Autodesk Inventor part; units mm, degrees
ref_plane "YZ Plane" through (0, 0, 0) normal (1, 0, 0) x (0, 1, 0)
ref_plane "XZ Plane" through (0, 0, 0) normal (0, 1, 0) x (-1, 0, 0)
ref_plane "XY Plane" through (0, 0, 0) normal (0, 0, 1) x (1, 0, 0)
ref_plane "Arbeitsebene1" through (-6.2499, 0, 0) normal (0, 0, 1) x (1, 0, 0)
sketch "Skizze1" plane through (-6.2499, 0, 0) normal (0, 0, 1) x (1, 0, 0)
  line L0 (21.2499, 26.0506) -> (21.2499, 58.2506)
  line L1 (21.2499, 58.2506) -> (-8.7501, 58.2506)
  line L2 (-8.7501, 58.2506) -> (-8.7501, 26.0506)
  line L3 (-8.7501, 26.0506) -> (21.2499, 26.0506)
  circle A0 centre (16.2499, 32.1506) radius 1.25
  circle A1 centre (-3.7501, 32.1506) radius 1.25
  circle A2 centre (-3.7501, 52.1506) radius 1.25
  circle A3 centre (16.2499, 52.1506) radius 1.25
  circle A4 centre (13.7499, 38.0506) radius 3.25
  circle A5 centre (13.7499, 46.2506) radius 3.25
  circle A6 centre (-1.2501, 38.0506) radius 3.25
  circle A7 centre (-1.2501, 46.2506) radius 3.25
  line L4 (-67.7501, 103.2266) -> (-67.7501, 101.9266) construction
  line L5 (-18.7501, 103.2266) -> (-67.7501, 103.2266) construction
  arc A8 (-15.2501, 99.7266) -> (-18.7501, 103.2266) centre (-18.7501, 99.7266) ccw construction
  line L6 (-15.2501, 22.1266) -> (-15.2501, 99.7266) construction
  arc A9 (-18.7501, 18.6266) -> (-15.2501, 22.1266) centre (-18.7501, 22.1266) ccw construction
  line L7 (-67.7501, 18.6266) -> (-18.7501, 18.6266) construction
  line L8 (-67.7501, 19.9266) -> (-67.7501, 18.6266) construction
  line L9 (-23.4028, 19.9266) -> (-67.7501, 19.9266) construction
  arc A10 (-23.4028, 19.9266) -> (-21.8472, 20.571) centre (-23.4028, 22.1266) ccw construction
  line L10 (-17.1945, 25.2237) -> (-21.8472, 20.571) construction
  arc A11 (-17.1945, 25.2237) -> (-16.5501, 26.7793) centre (-18.7501, 26.7793) ccw construction
  line L11 (-16.5501, 95.0739) -> (-16.5501, 26.7793) construction
  arc A12 (-16.5501, 95.0739) -> (-17.1945, 96.6296) centre (-18.7501, 95.0739) ccw construction
  line L12 (-21.8472, 101.2823) -> (-17.1945, 96.6296) construction
  arc A13 (-21.8472, 101.2823) -> (-23.4028, 101.9266) centre (-23.4028, 99.7266) ccw construction
  line L13 (-67.7501, 101.9266) -> (-23.4028, 101.9266) construction
  arc A14 (-18.7501, 18.2266) -> (-14.8501, 22.1266) centre (-18.7501, 22.1266) ccw construction
  line L14 (-14.8501, 22.1266) -> (-14.8501, 99.7266) construction
  line L15 (-18.7501, 103.6266) -> (-68.1501, 103.6266) construction
  line L16 (-68.1501, 103.6266) -> (-68.1501, 101.5266) construction
  line L17 (-68.1501, 101.5266) -> (-23.4028, 101.5266) construction
  arc A15 (-22.13, 100.9994) -> (-23.4028, 101.5266) centre (-23.4028, 99.7266) ccw construction
  line L18 (-22.13, 100.9994) -> (-17.4773, 96.3467) construction
  arc A16 (-16.9501, 95.0739) -> (-17.4773, 96.3467) centre (-18.7501, 95.0739) ccw construction
  line L19 (-16.9501, 95.0739) -> (-16.9501, 26.7793) construction
  arc A17 (-17.4773, 25.5065) -> (-16.9501, 26.7793) centre (-18.7501, 26.7793) ccw construction
  line L20 (-17.4773, 25.5065) -> (-22.13, 20.8538) construction
  arc A18 (-23.4028, 20.3266) -> (-22.13, 20.8538) centre (-23.4028, 22.1266) ccw construction
  line L21 (-23.4028, 20.3266) -> (-68.1501, 20.3266) construction
  line L22 (-68.1501, 20.3266) -> (-68.1501, 18.2266) construction
  line L23 (-68.1501, 18.2266) -> (-18.7501, 18.2266) construction
  arc A19 (-18.7501, 18.2266) -> (-14.8501, 22.1266) centre (-18.7501, 22.1266) ccw construction
  line L24 (-14.8501, 22.1266) -> (-14.8501, 99.7266) construction
  arc A20 (-14.8501, 99.7266) -> (-18.7501, 103.6266) centre (-18.7501, 99.7266) ccw construction
  line L25 (-89.5501, 101.9266) -> (-89.5501, 103.2266) construction
  line L26 (-138.8501, 101.9266) -> (-89.5501, 101.9266) construction
  arc A21 (-138.8501, 101.9266) -> (-140.7501, 100.0266) centre (-138.8501, 100.0266) ccw construction
  line L27 (-140.7501, 21.8266) -> (-140.7501, 100.0266) construction
  arc A22 (-140.7501, 21.8266) -> (-138.8501, 19.9266) centre (-138.8501, 21.8266) ccw construction
  line L28 (-89.5501, 19.9266) -> (-138.8501, 19.9266) construction
  line L29 (-89.5501, 18.6266) -> (-89.5501, 19.9266) construction
  line L30 (-138.5501, 18.6266) -> (-89.5501, 18.6266) construction
  arc A23 (-142.0501, 22.1266) -> (-138.5501, 18.6266) centre (-138.5501, 22.1266) ccw construction
  line L31 (-142.0501, 99.7266) -> (-142.0501, 22.1266) construction
  arc A24 (-138.5501, 103.2266) -> (-142.0501, 99.7266) centre (-138.5501, 99.7266) ccw construction
  line L32 (-89.5501, 103.2266) -> (-138.5501, 103.2266) construction
  arc A25 (-138.5501, 103.6266) -> (-142.4501, 99.7266) centre (-138.5501, 99.7266) ccw construction
  line L33 (-142.4501, 99.7266) -> (-142.4501, 22.1266) construction
  arc A26 (-142.4501, 22.1266) -> (-138.5501, 18.2266) centre (-138.5501, 22.1266) ccw construction
  line L34 (-138.5501, 18.2266) -> (-89.1501, 18.2266) construction
  line L35 (-89.1501, 18.2266) -> (-89.1501, 20.3266) construction
  line L36 (-89.1501, 20.3266) -> (-138.8501, 20.3266) construction
  arc A27 (-140.3501, 21.8266) -> (-138.8501, 20.3266) centre (-138.8501, 21.8266) ccw construction
  line L37 (-140.3501, 21.8266) -> (-140.3501, 100.0266) construction
  arc A28 (-138.8501, 101.5266) -> (-140.3501, 100.0266) centre (-138.8501, 100.0266) ccw construction
  line L38 (-138.8501, 101.5266) -> (-89.1501, 101.5266) construction
  line L39 (-89.1501, 101.5266) -> (-89.1501, 103.6266) construction
  line L40 (-89.1501, 103.6266) -> (-138.5501, 103.6266) construction
  line L41 (-68.6501, 104.1266) -> (-18.7501, 104.1266)
  arc A29 (-14.3501, 99.7266) -> (-18.7501, 104.1266) centre (-18.7501, 99.7266) ccw
  line L42 (-14.3501, 99.7266) -> (-14.3501, 22.1266)
  arc A30 (-18.7501, 17.7266) -> (-14.3501, 22.1266) centre (-18.7501, 22.1266) ccw
  line L43 (-18.7501, 17.7266) -> (-68.6501, 17.7266)
  line L44 (-68.6501, 17.7266) -> (-68.6501, 20.8266)
  line L45 (-68.6501, 20.8266) -> (-23.4028, 20.8266)
  arc A31 (-23.4028, 20.8266) -> (-22.4836, 21.2074) centre (-23.4028, 22.1266) ccw
  line L46 (-22.4836, 21.2074) -> (-17.8309, 25.8601)
  arc A32 (-17.8309, 25.8601) -> (-17.4501, 26.7793) centre (-18.7501, 26.7793) ccw
  line L47 (-17.4501, 26.7793) -> (-17.4501, 95.0739)
  arc A33 (-17.4501, 95.0739) -> (-17.8309, 95.9932) centre (-18.7501, 95.0739) ccw
  line L48 (-17.8309, 95.9932) -> (-22.4836, 100.6459)
  arc A34 (-22.4836, 100.6459) -> (-23.4028, 101.0266) centre (-23.4028, 99.7266) ccw
  line L49 (-23.4028, 101.0266) -> (-68.6501, 101.0266)
  line L50 (-68.6501, 101.0266) -> (-68.6501, 104.1266)
  arc A35 (-138.5501, 104.1266) -> (-142.9501, 99.7266) centre (-138.5501, 99.7266) ccw
  line L51 (-142.9501, 99.7266) -> (-142.9501, 22.1266)
  arc A36 (-142.9501, 22.1266) -> (-138.5501, 17.7266) centre (-138.5501, 22.1266) ccw
  line L52 (-138.5501, 17.7266) -> (-88.6501, 17.7266)
  line L53 (-88.6501, 17.7266) -> (-88.6501, 20.8266)
  line L54 (-88.6501, 20.8266) -> (-138.8501, 20.8266)
  arc A37 (-139.8501, 21.8266) -> (-138.8501, 20.8266) centre (-138.8501, 21.8266) ccw
  line L55 (-139.8501, 21.8266) -> (-139.8501, 100.0266)
  arc A38 (-138.8501, 101.0266) -> (-139.8501, 100.0266) centre (-138.8501, 100.0266) ccw
  line L56 (-138.8501, 101.0266) -> (-88.6501, 101.0266)
  line L57 (-88.6501, 101.0266) -> (-88.6501, 104.1266)
  line L58 (-88.6501, 104.1266) -> (-138.5501, 104.1266)
  line L59 (-68.6501, 104.1266) -> (-88.6501, 104.1266)
  line L60 (-88.6501, 17.7266) -> (-68.6501, 17.7266)
  line L61 (-94.9, 12.7266) -> (-138.5501, 12.7266)
  arc A39 (-147.9501, 22.1266) -> (-138.5501, 12.7266) centre (-138.5501, 22.1266) ccw
  line L62 (-147.9501, 22.1266) -> (-147.9501, 99.7266)
  arc A40 (-138.5501, 109.1266) -> (-147.9501, 99.7266) centre (-138.5501, 99.7266) ccw
  line L63 (-138.5501, 109.1266) -> (-94.9, 109.1266)
  line L64 (-74.9, 12.7266) -> (-18.7501, 12.7266)
  arc A41 (-18.7501, 12.7266) -> (-9.3501, 22.1266) centre (-18.7501, 22.1266) ccw
  line L65 (-9.3501, 22.1266) -> (-9.3501, 99.7266)
  arc A42 (-9.3501, 99.7266) -> (-18.7501, 109.1266) centre (-18.7501, 99.7266) ccw
  line L66 (-18.7501, 109.1266) -> (-74.9, 109.1266)
  line L67 (-94.9, 12.7266) -> (-74.9, 12.7266)
  line L68 (-74.9, 109.1266) -> (-94.9, 109.1266)
  line L69 (-8.7501, 58.2506) -> (-9.3501, 58.2506)
  line L70 (-8.7501, 26.0506) -> (-9.3501, 26.0506)
  point P0 (6.2499, 0)
  point P1 (-12.4751, 58.2506)
  point P2 (-12.4751, 26.0506)
  point P3 (-12.4751, 26.0506)
  dimension "d0" = 0
  dimension "d1" = 0
  dimension "d2" = 0.5
  dimension "d3" = 0.5
  dimension "d4" = 5
  dimension "d5" = 5
extrude "Extrusion1" add sketch "Skizze1" along normal blind 10 contours L3 L2 L1 L0 | L70 L65 L69 L2 | L65 A41 L64 L67 L61 A39 L62 A40 L63 L68 L66 A42 | A4 | A5 | A6 | A7
sketch "Skizze3" plane through (-6.2499, 0, 0) normal (0, 0, -1) x (-1, 0, 0)
  line L0 (9.3501, 26.0506) -> (-21.2499, 26.0506)
  line L1 (9.3501, 22.1266) -> (9.3501, 26.0506)
  arc A0 (9.3501, 22.1266) -> (18.7501, 12.7266) centre (18.7501, 22.1266) ccw
  line L2 (138.5501, 12.7266) -> (18.7501, 12.7266)
  arc A1 (138.5501, 12.7266) -> (147.9501, 22.1266) centre (138.5501, 22.1266) ccw
  line L3 (147.9501, 99.7266) -> (147.9501, 22.1266)
  arc A2 (147.9501, 99.7266) -> (138.5501, 109.1266) centre (138.5501, 99.7266) ccw
  line L4 (18.7501, 109.1266) -> (138.5501, 109.1266)
  arc A3 (18.7501, 109.1266) -> (9.3501, 99.7266) centre (18.7501, 99.7266) ccw
  line L5 (9.3501, 58.2506) -> (9.3501, 99.7266)
  line L6 (-21.2499, 58.2506) -> (9.3501, 58.2506)
  line L7 (-21.2499, 26.0506) -> (-21.2499, 58.2506)
  circle A4 centre (-16.2499, 32.1506) radius 1.25
  circle A5 centre (3.7501, 32.1506) radius 1.25
  circle A6 centre (3.7501, 52.1506) radius 1.25
  circle A7 centre (-16.2499, 52.1506) radius 1.25
  line L8 (18.7501, 17.7266) -> (138.5501, 17.7266)
  arc A8 (14.3501, 22.1266) -> (18.7501, 17.7266) centre (18.7501, 22.1266) ccw
  line L9 (14.3501, 99.7266) -> (14.3501, 22.1266)
  arc A9 (18.7501, 104.1266) -> (14.3501, 99.7266) centre (18.7501, 99.7266) ccw
  line L10 (138.5501, 104.1266) -> (18.7501, 104.1266)
  arc A10 (142.9501, 99.7266) -> (138.5501, 104.1266) centre (138.5501, 99.7266) ccw
  line L11 (142.9501, 22.1266) -> (142.9501, 99.7266)
  arc A11 (138.5501, 17.7266) -> (142.9501, 22.1266) centre (138.5501, 22.1266) ccw
  arc A12 (141.4501, 99.7266) -> (138.5501, 102.6266) centre (138.5501, 99.7266) ccw
  line L12 (138.5501, 102.6266) -> (18.7501, 102.6266)
  arc A13 (18.7501, 102.6266) -> (15.8501, 99.7266) centre (18.7501, 99.7266) ccw
  line L13 (15.8501, 99.7266) -> (15.8501, 22.1266)
  arc A14 (15.8501, 22.1266) -> (18.7501, 19.2266) centre (18.7501, 22.1266) ccw
  line L14 (18.7501, 19.2266) -> (138.5501, 19.2266)
  arc A15 (138.5501, 19.2266) -> (141.4501, 22.1266) centre (138.5501, 22.1266) ccw
  line L15 (141.4501, 22.1266) -> (141.4501, 99.7266)
  point P0 (-6.2499, 0)
  dimension "d11" = 1.5
extrude "Extrusion3" add sketch "Skizze3" against normal blind 1 contours A8 L9 A9 L10 A10 L11 A11 L8
sketch "Skizze4" plane through (-144.8, 12.7266, 0) normal (0, -1, 0) x (1, 0, 0)
  line L0 (0, 10) -> (119.8, 10)
  line L1 (19.9, 10) -> (99.9, 10) construction
  line L2 (0, 10) -> (119.8, 10)
  line L3 (19.9, 7.5) -> (99.9, 7.5)
  line L4 (99.9, 12.5) -> (19.9, 12.5)
  arc A0 (19.9, 12.5) -> (19.9, 7.5) centre (19.9, 10) ccw
  arc A1 (99.9, 7.5) -> (99.9, 12.5) centre (99.9, 10) ccw
  point P0 (144.8, 0)
  point P1 (59.9, 10)
  point P2 (102.4, 10)
  point P3 (17.4, 10)
  dimension "d14" = 40
  dimension "d18" = 5
extrude "Extrusion4" cut sketch "Skizze4" against normal through all contours L0 A1 L3 A0
fillet "Rundung1" radius 2 4 edges at (-127.4, 15.2266, 10) (-127.4, 106.6266, 10) (-42.4, 106.6266, 10) (-42.4, 15.2266, 10)
properties part number "20_Cube_Insert_Linear_Stage_NEMA11_china_wellplatemount"
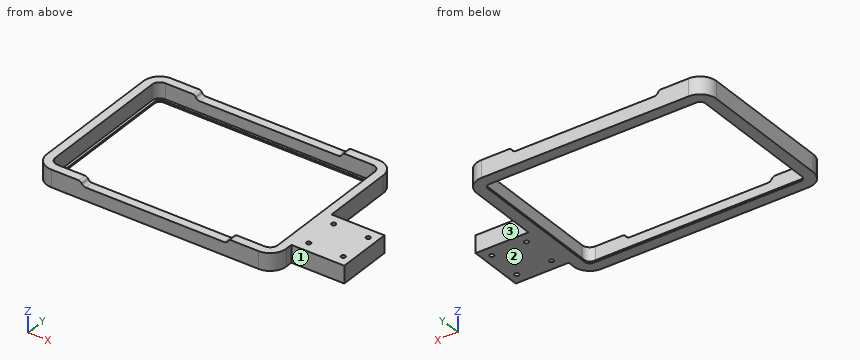
Check sheet for the modelled part. Datum: model origin and axes. Units: mm. Face numbers are marked on the shaded views. A direction names the side the tool comes from. Round coordinates to 2 decimals unless told otherwise and drop trailing zeros. Loops run counter-clockwise (first coordinate to the right, second up) from the corner with the lowest first, then second, coordinate; pieces in that order, holes last. Notation, with made-up numbers: (77, 59) - (105, 59) arc R17 ccw to (105, 80) - close; hole circle Ø1 at (56.5, 43.5). An arc over 180 degrees is marked (long way). Answer as CSV lines item,"result". Start each with the question number.
Item 1: Set-up check for the marked faces 1, 2 and 3: record each of +Z, -Z, +X, -X, +Y, -Y from which the full face is reachable in a straight line by a thin tool's end or side.
Item 2: Section check B-B (y = 36). Record the boundary of the cut face in (x, z), and give its area (3 significant figures).
Item 3: Depth check by flat-ended pin: P1, Ø5, axis at x = 6, z = 5.5, coming from the +Y side; P2, Ø1, axis at y = 82.5, z = 4.5, coming from the +X side; P3, Ø2.5, axis at x = -69, y = 15.5, coming from the +Z side. Enter the tip coordinate at first touch or a pass-through.
Item 4: Section check A-A (x = -142.5). Record the boundary of the cut face in (y, z), and give its area (3 significant figures).
Item 5: Scan lines: line 1 (Y direction, x = -10, z = 7); line 2 (X direction, y = 57, z = 7.5); line 3 (X direction, y = 72, z = 9). Record each from-to range of solid material in increasing order. Write a range as [from, to].
Item 6: Section check D-D (x = -13.5). Record the boundary of the cut face in (y, z), and give its area (3 significant figures).
Item 7: Section check C-C (z = 4.75). Record the boundary of the cut face in (x, y).
Report:
1,face 1,"+Z, -Z, +X, -Y"
1,face 2,"-Z, +X, -X, +Y, -Y"
1,face 3,"+Z, -Z, +X, +Y"
2,outline,"(-154.2, 0) - (-147.7, 0) - (-147.7, 1) - (-149.2, 1) - (-149.2, 10) - (-154.2, 10) - close; (-22.1, 0) - (15, 0) - (15, 10) - (-20.6, 10) - (-20.6, 1) - (-22.1, 1) - close"
2,area,"409 mm2"
3,P1,"stops at y = 58.25"
3,P2,"stops at x = -15.6"
3,P3,"stops at z = 7.5"
4,outline,"(12.73, 0) - (19.23, 0) - (19.23, 1) - (17.73, 1) - (17.73, 10) - (12.73, 10) - close; (102.63, 0) - (109.13, 0) - (109.13, 10) - (104.13, 10) - (104.13, 1) - (102.63, 1) - close"
4,area,"103 mm2"
5,line 1,"y = [26.05, 30.9], [33.4, 50.9], [53.4, 58.25]"
5,line 2,"x = [-154.2, -149.2], [-20.6, 15]"
5,line 3,"x = [-154.2, -149.2], [-20.6, -15.6]"
6,outline,"(26.05, 0) - (58.25, 0) - (58.25, 10) - (26.05, 10) - close"
6,area,"322 mm2"
7,outline,"(-154.2, 22.13) arc R9.4 ccw to (-144.8, 12.73) - (-25, 12.73) arc R9.4 ccw to (-15.6, 22.13) - (-15.6, 26.05) - (15, 26.05) - (15, 58.25) - (-15.6, 58.25) - (-15.6, 99.73) arc R9.4 ccw to (-25, 109.13) - (-144.8, 109.13) arc R9.4 ccw to (-154.2, 99.73) - close; hole (-149.2, 22.13) arc R4.4 ccw to (-144.8, 17.73) - (-25, 17.73) arc R4.4 ccw to (-20.6, 22.13) - (-20.6, 99.73) arc R4.4 ccw to (-25, 104.13) - (-144.8, 104.13) arc R4.4 ccw to (-149.2, 99.73) - close; hole circle Ø2.5 at (-10, 32.15); hole circle Ø2.5 at (-10, 52.15); hole circle Ø2.5 at (10, 32.15); hole circle Ø2.5 at (10, 52.15)"
